Source: CAD feature listing. Evaluate the final solid. Frame: model axes, mm. A direction names the side the tool comes from. Coordinates: 2 decimals unless noted, no trailing zeros. Write each loop counter-clockwise with the first axis right and the second up, starting at its lowest first coordinate (ties: lowest second). Pieces come first, ordered by that corner, then holes. Notation, with made-up numbers: (77.25, 23) - (92.25, 23) arc R16 cw to (92.25, 41) - close; hole circle Ø6 at (67.5, -26.5). An arc over 180 degrees is marked (long way). One line per question, with ' | ' between items. Start each with the question number.
Q1. Draft query along Y for faces 1 (the face through (10.9, 5, 2)), 2 (the face through (8, 4, -4)). Return one class per face: +Y half, -Y half, draft (parallel to the pull), parting line (faces both ways), or undercut.
Q2. Access query for faces 3 (the face through (0, 6, 7)), 4 (the face through (3.944, -7.167, -4.57)). Directions: +Z, -Z, +X, -X, +Y, -Y. A direction counts if a zero-diameter tool reaches every point of the face in a straight line with its end or side. Return the directions, or none.
Q3. Contact query for flat-ended pins moving along their axis: P1, Ø2, axis at y = 10, z = -11.5, coming from the -X side; P2, Ø4, axis at x = 5.5, z = 6, coming from the +Y side; P3, Ø5, axis at y = 8, z = 1, coming from the -X side; P4, Ø16, axis at y = 0, z = 0, coming from the -X side. Output: stop coordinate, or through.
Q4. Cut plane A-A, the plane y = 0. Return loops of the section in (x, z).
Q5. Cut plane D-D, the plane x = 3. Return loops of the section in (y, z), plus the area to 3 significant figures.
Q6. Cut plane C-C, the plane x = 1. Return loops of the section in (y, z), plus the area to 3 significant figures.
Q7. Line query: line 1 (Z direction, x = 2.5, y = 6); line 2 (Z direction, x = 4.75, y = 0); line 3 (X direction, y = 3, z = -7.5). Output: solid intervals per line, ascending.
```python
from build123d import *

# Parameters (mm, degrees)
SKETCH010_R     = 8.5
POCKET005_DEPTH = 8
SKETCH011_R     = 5
POCKET006_DEPTH = 10.901


with BuildPart() as part:
    # Sketch009 → Revolution002 (revolve)
    with BuildSketch(Plane.XZ):
        with BuildLine():
            Line((0, 0), (0, 10.9))
            Line((0, 10.9), (0.3, 10.9))
            Line((0.3, 10.9), (0.3, 15))
            Line((0.3, 15), (0.5, 15))
            ThreePointArc((0.5, 15), (5.310502, 11.962006), (10.9, 10.9))
            Line((10.9, 10.9), (10.9, 0))
            Line((10.9, 0), (0, 0))
        make_face()
    revolve(axis=Axis((0, 0, 0), (1, 0, 0)))

    # Sketch010 (on Face1 of Revolution002) → Pocket005 (cut)
    with BuildSketch(Plane(origin=(0, 0, 0), x_dir=(0, 0, -1), z_dir=(-1, 0, 0))):
        Circle(SKETCH010_R)
    extrude(amount=-POCKET005_DEPTH, mode=Mode.SUBTRACT)

    # Sketch011 (on Face8 of Pocket005) → Pocket006 (cut, through all)
    with BuildSketch(Plane(origin=(10.9, 0, 0), x_dir=(0, 0, 1), z_dir=(1, 0, 0))):
        Circle(SKETCH011_R)
    extrude(amount=-POCKET006_DEPTH, mode=Mode.SUBTRACT)


solid = part.part
```
Reply:
1) face 1: draft | face 2: undercut
2) face 3: +Z, -Z, -X, +Y, -Y | face 4: -X
3) P1: stops at x = 0.3 | P2: stops at y = 11.65 | P3: stops at x = 0 | P4: stops at x = 8
4) outline: (0, -10.9) - (0.3, -10.9) - (0.3, -15) - (0.5, -15) arc R15.24 cw to (10.9, -10.9) - (10.9, -5) - (8, -5) - (8, -8.5) - (0, -8.5) - close; (0, 8.5) - (8, 8.5) - (8, 5) - (10.9, 5) - (10.9, 10.9) arc R15.24 cw to (0.5, 15) - (0.3, 15) - (0.3, 10.9) - (0, 10.9) - close
5) outline: circle Ø26.21 at (0, 0); hole circle Ø17 at (0, 0) | area: 313 mm^2
6) outline: circle Ø29.11 at (0, 0); hole circle Ø17 at (0, 0) | area: 438 mm^2
7) line 1: z = -12.01 to -6.02, 6.02 to 12.01 | line 2: z = -12.2 to -8.5, 8.5 to 12.2 | line 3: x = 8 to 10.9
